```python
from build123d import *

# Parameters (mm, degrees)
SKETCH1_W      = 18
SKETCH1_H      = 27
SKETCH1_R      = 2.5
EXTRUDE1_DEPTH = 0.5
SKETCH2_W      = 18
SKETCH2_H      = 0.5
EXTRUDE2_DEPTH = 8.9
SKETCH3_R      = 1.5
EXTRUDE3_DEPTH = 0.5
SKETCH4_R      = 1.5
EXTRUDE4_DEPTH = 0.5


with BuildPart() as part:
    # Sketch1 → Extrude1 (new body)
    with BuildSketch(Plane.XY):
        with Locations((0, -6.5)):
            Rectangle(SKETCH1_W, SKETCH1_H)
        Circle(SKETCH1_R, mode=Mode.SUBTRACT)
    extrude(amount=EXTRUDE1_DEPTH)

    # Sketch2 → Extrude2 (add)
    with BuildSketch(Plane(origin=(0, 0, 0), x_dir=(-1, 0, 0), z_dir=(0, 0, -1))):
        with Locations((0, -19.75)):
            Rectangle(SKETCH2_W, SKETCH2_H)
    extrude(amount=EXTRUDE2_DEPTH)

    # Sketch3 → Extrude3 (cut)
    with BuildSketch(Plane(origin=(0, -19.5, 0), x_dir=(1, 0, 0), z_dir=(0, 1, 0))):
        with Locations(Location((-5, 5.9, 0), (0, 0, 180))):
            Circle(SKETCH3_R)
        with Locations(Location((5, 5.9, 0), (0, 0, 180))):
            Circle(SKETCH3_R)
    extrude(amount=-EXTRUDE3_DEPTH, mode=Mode.SUBTRACT)

    # Sketch4 → Extrude4 (cut)
    with BuildSketch(Plane(origin=(0, 0, 0), x_dir=(-1, 0, 0), z_dir=(0, 0, -1))):
        with Locations((-6.443229004, -3.72)):
            Circle(SKETCH4_R)
        with Locations((6.443229004, 3.72)):
            Circle(SKETCH4_R)
    extrude(amount=-EXTRUDE4_DEPTH, mode=Mode.SUBTRACT)


solid = part.part
```
Geometry: final body of the model. Coordinates: model frame, mm. A direction names the side the tool comes from. Round coordinates to 2 decimals unless told otherwise and drop trailing zeros. Order: outer loops, then holes, each group sorted by start corner. A loop starts at its lowest first (then second) coordinate and runs counter-clockwise, first axis right, second up. Notation, with made-up numbers: M 4,20 L 58,20 A11 ccw 58,33 Z; hole C -11,-24.5 d3. An arc over 180 degrees is marked long. One line per item, written item: value.
(1) Reachability of faces 1 (the cylindrical face through (6.5, -19.75, -5.83)), 2 (the flat face through (0, -19.5, -4)) from +Z, -Z, +X, -X, +Y, -Y: full face, straight path, thin tool, end or side. Return the list, or none.
Result sheet:
face 1: +Y, -Y
face 2: -Z, +X, -X, +Y
(2) Pull-direction query (X, two-part tool) for faces 3 (the flat face through (0, -6, 0.5)), 4 (the flat face through (-9, -12.6, 0.3)), 5 (the cylindrical face through (-6.118, 2.256, 0.246)); classes: pulls with the +X half, pulls with the -X half, needs draft (parallel to the pull), parting line crosses it, or undercut.
Result sheet:
face 3: needs draft
face 4: pulls with the -X half
face 5: undercut
(3) Cut plane D-D (x = 6). Return the cut outline in (y, z).
Result sheet:
outline: M -20,-8.9 L -19.5,-8.9 L -19.5,-7.02 L -20,-7.02 Z; M -20,-4.78 L -19.5,-4.78 L -19.5,0 L -5.15,0 L -5.15,0.5 L -20,0.5 Z; M -2.29,0 L 7,0 L 7,0.5 L -2.29,0.5 Z
(4) Cut plane A-A (y = 0). Return the cut outline in (x, z), and give its area (3 significant figures).
Result sheet:
outline: M -9,0 L -2.5,0 L -2.5,0.5 L -9,0.5 Z; M 2.5,0 L 9,0 L 9,0.5 L 2.5,0.5 Z
area: 6.50 mm2
(5) Pin query (flat end, axial travel): P1, Ø3.5, axis at x = -5, z = -5.9, coming from the +Y side; P2, Ø5.5, axis at x = 4, y = -2, coming from the -Z side; P3, Ø4.5, axis at x = 0, y = 0, coming from the -Z side. Return the tip coordinate at first contact, or that it passes through.
Result sheet:
P1: y = -19.5
P2: z = 0
P3: through
(6) Cut plane C-C (x = -2). Return the cut outline in (y, z).
Result sheet:
outline: M -20,-8.9 L -19.5,-8.9 L -19.5,0 L -1.5,0 L -1.5,0.5 L -20,0.5 Z; M 1.5,0 L 7,0 L 7,0.5 L 1.5,0.5 Z
(7) Line query: probe 1 along Z at (x, y) = (-5, -19.75); probe 2 along Y at (x, z) = (-5.5, -1.5); probe 3 along Z at (x, y) = (3.5, -18.75). Output: solid intervals per line, ascending. Write a range as [from, to].
Result sheet:
probe 1: [-8.9, -7.4], [-4.4, 0.5]
probe 2: [-20, -19.5]
probe 3: [0, 0.5]
(8) Cut plane B-B (z = -5.9). Return the cut outline in (x, y), and give its area (3 significant figures).
Result sheet:
outline: M -9,-20 L -6.5,-20 L -6.5,-19.5 L -9,-19.5 Z; M -3.5,-20 L 3.5,-20 L 3.5,-19.5 L -3.5,-19.5 Z; M 6.5,-20 L 9,-20 L 9,-19.5 L 6.5,-19.5 Z
area: 6.00 mm2
